Verification items for the finished model (mm, model axes). A direction names the side the tool comes from. Coordinates: 2 decimals unless noted, no trailing zeros. Write each loop counter-clockwise with the first axis right and the second up, starting at its lowest first coordinate (ties: lowest second). Pieces come first, ordered by that corner, then holes. Notation, with made-up numbers: M -4.75,84 L -0.75,84 A29 cw -0.75,118 Z; hole C 78,-5.75 d2. An arc over 180 degrees is marked long. One line per item, written item: value.
```python
from build123d import *

# Parameters (mm, degrees)
BOSS_EXTRUDE1_DEPTH = 5
SKETCH3_W           = 63
SKETCH3_H           = 27
BOSS_EXTRUDE3_DEPTH = 2.5
SKETCH4_R           = 1
BOSS_EXTRUDE6_DEPTH = 4
SKETCH5_W           = 1
SKETCH5_H           = 3.04418771
CUT_EXTRUDE1_DEPTH  = 3
SKETCH6_R           = 1.15
BOSS_EXTRUDE7_DEPTH = 1
CHAMFER1_SIZE       = 0.5
SKETCH7_W           = 1
SKETCH7_H           = 2.786400566
CUT_EXTRUDE3_DEPTH  = 1
MIRROR2_START       = 47
MIRROR2_DEPTH       = 1


with BuildPart() as part:
    # Sketch1 → Boss-Extrude1 (new, symmetric)
    with BuildSketch(Plane.XY):
        Polygon((0, 0), (10, 0), (40, 2.624659906), (39.566186352, 7.583172591), (10, 4.996466462), (5, 4.996466462), (5, 38.996466462), (50, 38.996466462), (50, 43), (0, 43), align=None)
    extrude(amount=BOSS_EXTRUDE1_DEPTH, both=True)

    # Sketch3 → Boss-Extrude3 (add, symmetric)
    with BuildSketch(Plane(origin=(0, 40.5, 0), x_dir=(1, 0, 0), z_dir=(0, 1, 0))):
        with Locations((31.5, 8.5)):
            Rectangle(SKETCH3_W, SKETCH3_H)
    extrude(amount=BOSS_EXTRUDE3_DEPTH, both=True)

    # Sketch4 → Boss-Extrude6 (add)
    with BuildSketch(Plane(origin=(0, 43, 0), x_dir=(1, 0, 0), z_dir=(0, 1, 0))):
        with Locations(Location((2, -1, 0), (0, 0, 90))):
            Circle(SKETCH4_R)
        with Locations(Location((2, 18, 0), (0, 0, 90))):
            Circle(SKETCH4_R)
    extrude(amount=BOSS_EXTRUDE6_DEPTH)

    # Sketch5 → Cut-Extrude1 (cut)
    with BuildSketch(Plane(origin=(0, 47, 0), x_dir=(1, 0, 0), z_dir=(0, 1, 0))):
        with Locations((2, -1)):
            Rectangle(SKETCH5_W, SKETCH5_H)
    cut_extrude1 = extrude(amount=-CUT_EXTRUDE1_DEPTH, mode=Mode.SUBTRACT)

    # Mirror1: Cut-Extrude1 across plane
    add(cut_extrude1.mirror(Plane.XY.offset(-8.5)), mode=Mode.SUBTRACT)

    # Sketch6 → Boss-Extrude7 (add)
    with BuildSketch(Plane(origin=(0, 47, 0), x_dir=(1, 0, 0), z_dir=(0, 1, 0))):
        with Locations(Location((2, -1, 0), (0, 0, 270))):
            Circle(SKETCH6_R)
    extrude(amount=BOSS_EXTRUDE7_DEPTH)

    # Chamfer1
    chamfer1_edges = [part.edges().sort_by_distance(p)[0] for p in [
        (2, 48, -0.15),
    ]]
    chamfer(chamfer1_edges, length=CHAMFER1_SIZE)

    # Sketch7 → Cut-Extrude3 (cut)
    with BuildSketch(Plane(origin=(0, 48, 0), x_dir=(1, 0, 0), z_dir=(0, 1, 0))):
        with Locations((2, -1)):
            Rectangle(SKETCH7_W, SKETCH7_H)
    extrude(amount=-CUT_EXTRUDE3_DEPTH, mode=Mode.SUBTRACT)

    # Mirror2: read off the stored shape, not the designer's step
    # Mirror2 outline → Mirror2 (add)
    with BuildSketch(Plane(origin=(0, 0, 0), x_dir=(1, 0, 0), z_dir=(0, 1, 0)).offset(MIRROR2_START)):
        with BuildLine():
            ThreePointArc((2.5, 16.964384241), (3.15, 18), (2.5, 19.035615759))
            Line((2.5, 19.035615759), (2.5, 16.964384241))
        make_face()
        with BuildLine():
            ThreePointArc((1.5, 19.035615759), (0.85, 18), (1.5, 16.964384241))
            Line((1.5, 16.964384241), (1.5, 19.035615759))
        make_face()
    extrude(amount=MIRROR2_DEPTH)

    # Mirror2 2 outline → Mirror2 2 (revolve, cut)
    with BuildSketch(Plane(origin=(2, 0, -18), x_dir=(1, 0, 0), z_dir=(0, 0, 1))):
        Polygon((1.150000012, 48.000000304), (0.649999696, 48.000000304), (1.150000012, 47.499999988), align=None)
    revolve(axis=Axis((2, 0, -18), (0, 1, 0)), mode=Mode.SUBTRACT)


solid = part.part
```
Item 1: Cross-section at A-A, the plane x = 22.5. Enter the section's corners in (y, z), and give its area (3 significant figures).
The answers:
outline: M 1.09,-5 L 6.09,-5 L 6.09,5 L 1.09,5 Z; M 38,-22 L 43,-22 L 43,5 L 38,5 Z
area: 185 mm²
Item 2: Scan lines: line 1 (Y direction, x = 8.5, z = -0.75); line 2 (X direction, y = 22.5, z = -2.5); line 3 (Y direction, x = 46.5, z = -10.75). Record each from-to range of solid material in increasing order.
The answers:
line 1: y = 0 to 5, 38 to 43
line 2: x = 0 to 5
line 3: y = 38 to 43
Item 3: Go/stop test with flat-tipped pins: P1, Ø3, axis at x = 16.5, z = -5, coming from the -Y side; P2, Ø2.5, axis at y = 46.5, z = -18, coming from the -X side; P3, Ø5, axis at x = 48, z = -16, coming from the +Y side. Record where each tip stops, or that it passes through.
The answers:
P1: stops at y = 0.44
P2: stops at x = 0.85
P3: stops at y = 43
Item 4: Draft check along Z on faces 1 (the face through (1.324, 44.972, 1.737)), 2 (the face through (15, 5, -5)), 3 (the face through (2.5, 46, 1)). Enter one of: released by +Z, released by -Z, zero draft, split by the parting line, or undercut.
The answers:
face 1: undercut
face 2: released by -Z
face 3: zero draft
Item 5: Access from +Z, -Z, +X, -X, +Y, -Y to the whole of each face (thin tool, end or side, straight path). Record for faces 4 (the face through (8, 4.996, 0)), 5 (the face through (39.786, 5.069, 0.07)), 6 (the face through (2.5, 46, -18)), 7 (the face through (1.324, 44.972, -17.263)), 8 (the face through (63, 41, -8)).
The answers:
face 4: +Z, -Z
face 5: +Z, -Z, +X
face 6: +Z, -Z, +Y
face 7: none
face 8: +Z, -Z, +X, +Y, -Y
Item 6: Cross-section at B-B, the plane z = -11.75. Enter the section's corners in (x, y), and give its area (3 significant figures).
The answers:
outline: M 0,38 L 63,38 L 63,43 L 0,43 Z
area: 315 mm²
Item 7: Cross-section at C-C, the plane x = 52.5. Enter the section's corners in (y, z).
The answers:
outline: M 38,-22 L 43,-22 L 43,5 L 38,5 Z
